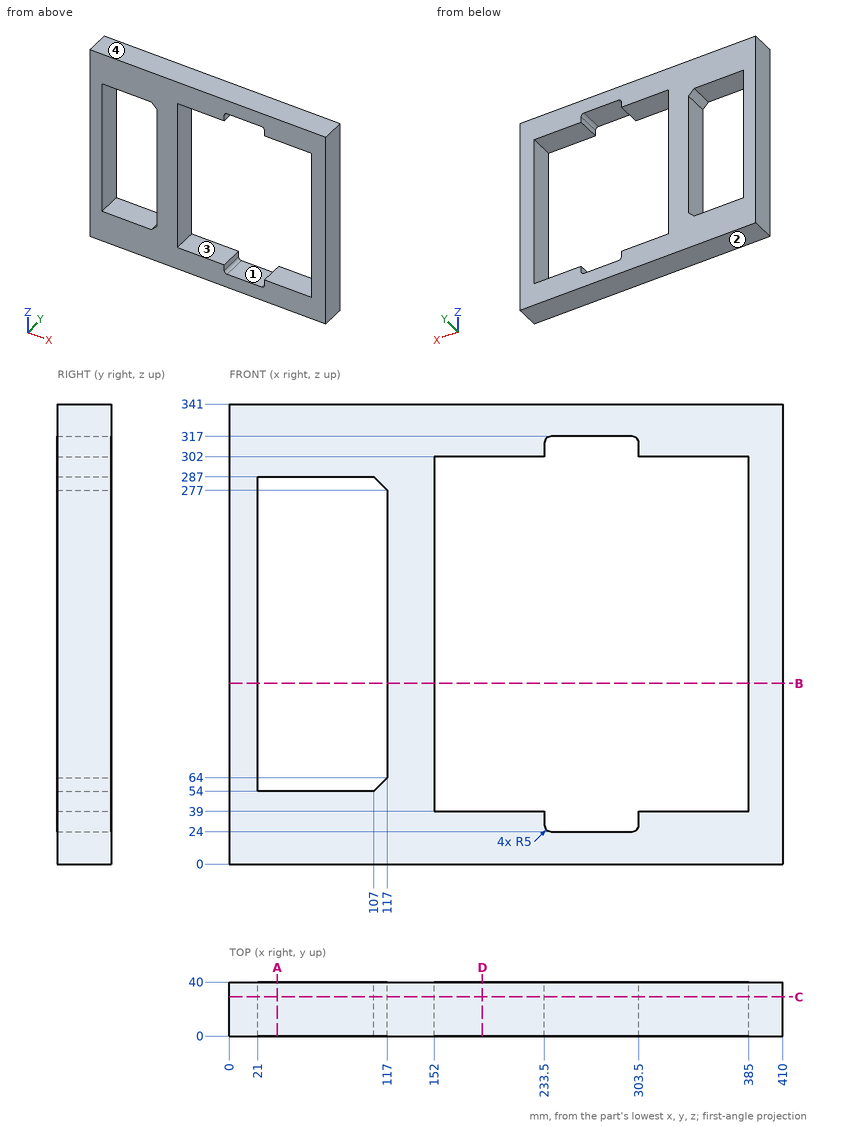
Here's the drawing with two shaded views (mm, measured from the low corner). I have some questions. A direction names the side the tool comes from. Coordinates: 2 decimals unless noted, no trailing zeros. Loops run counter-clockwise (first coordinate to the right, second up) from the corner with the lowest first, then second, coordinate; pieces in that order, holes last.
Item 1: Please list where these lines run through material, in increasing order: L1, parallel to X at y = 36, z = 257; L2, parallel to Z at x = 228, y = 22.5; L3, parallel to X at y = 12.5, z = 38.5.
Answers below:
L1: x = 0 to 21, 117 to 152, 385 to 410
L2: z = 0 to 39, 302 to 341
L3: x = 0 to 233.5, 303.5 to 410
Item 2: Which directions (+Z, -Z, +X, -X, +Y, -Y) give clear straight access to the entire face, cutting with the end or side of a thin tool? Please do the marked faces 1 and 2.
Answers below:
face 1: +Y, -Y
face 2: -Z, +X, -X, +Y, -Y
Item 3: Suppose I cut it at A-A (x = 35.5). Please give me the cut outline in (y, z).
Answers below:
outline: (0, 0) - (40, 0) - (40, 54) - (0, 54) - close; (0, 287) - (40, 287) - (40, 341) - (0, 341) - close
Item 4: Suppose I cut it at B-B (z = 134). Please give me the cut outline in (x, y), then the cut area to 3 significant figures.
Answers below:
outline: (0, 0) - (21, 0) - (21, 40) - (0, 40) - close; (117, 0) - (152, 0) - (152, 40) - (117, 40) - close; (385, 0) - (410, 0) - (410, 40) - (385, 40) - close
area: 3,240 mm2
Item 5: If we mould it in two halves opening along X, with no side actions, what happens to the marked faces 3 and 4? For each: released by +X, released by -X, zero draft, split by the parting line, or undercut.
Answers below:
face 3: undercut
face 4: zero draft
Item 6: Suppose I cut it at C-C (y = 29). Please give me the cut outline in (x, z), then the cut area to 3 significant figures.
Answers below:
outline: (0, 0) - (410, 0) - (410, 341) - (0, 341) - close; hole (21, 54) - (107, 54) - (117, 64) - (117, 277) - (107, 287) - (21, 287) - close; hole (152, 39) - (233.5, 39) - (233.5, 29) arc R5 ccw to (238.5, 24) - (298.5, 24) arc R5 ccw to (303.5, 29) - (303.5, 39) - (385, 39) - (385, 302) - (303.5, 302) - (303.5, 312) arc R5 ccw to (298.5, 317) - (238.5, 317) arc R5 ccw to (233.5, 312) - (233.5, 302) - (152, 302) - close
area: 54,200 mm2
Item 7: Suppose I cut it at D-D (x = 187.5). Please give me the cut outline in (y, z).
Answers below:
outline: (0, 0) - (40, 0) - (40, 39) - (0, 39) - close; (0, 302) - (40, 302) - (40, 341) - (0, 341) - close
